Read the model definition and answer for the solid it produces. Units are mm, in the model's axes. A direction names the side the tool comes from. Coordinates: 2 decimals unless noted, no trailing zeros. Loops run counter-clockwise (first coordinate to the right, second up) from the corner with the lowest first, then second, coordinate; pieces in that order, holes last. Notation, with made-up numbers: (79.25, 29.25) -> (117.25, 29.25) arc R21 ccw to (117.25, 68.25) -> close; hole circle Ø7 at (-7, 74.5). An arc over 180 degrees is marked (long way). Answer as a JSON object with one key per item and string values. Group by question number.
Q1. The part is cut by section B-B on y = 0. Write down the section's boundary in (x, z).
Q2. The part is cut by section A-A on z = 4.3. Write down the section's boundary in (x, y).
Q3. For faces 1 (the flat face through (-9.754, 0, 4)), 2 (the cylindrical face through (-2.256, 0.154, 2.958)), determine the directions among +Z, -Z, +X, -X, +Y, -Y from which every point of the face is accessible in a straight line to the end or side of a thin tool.
Q4. Straight lines are drawn through the part: line 1 along Z through (x, y) = (-12.5, -1.5); line 2 along X through (y, z) = (4.25, 4.9); line 3 along X through (y, z) = (-3, 3.55). For each, find the intervals that lie inside material, in ascending order. Write a range as [from, to].
Q5. The part is cut by section D-D on y = 2.75. Write down the section's boundary in (x, z).
Q6. Determine the mould class of faces 3 (the cylindrical face through (-34.252, -0.154, 2.958)), 4 (the flat face through (-25.821, -5.446, 4.028)), 5 (the flat face through (-24, 0, 2)), 6 (the flat face through (-18.4, 7, 1.6)) for opening direction X: released by +X, released by -X, zero draft, split by the parting line, or undercut.
Q7. Each of these flat-tipped pins is pushed along its axis until it touches: P1, Ø1.5, axis at y = 5.5, z = 4, coming from the -X side; P2, Ø3, axis at y = 4.5, z = 4.5, coming from the -X side; P3, Ø1, axis at y = -2.5, z = 3, coming from the -X side. Where does it stop, or does it pass through?
Q8. The part is cut by section C-C on z = 1.25. Write down the section's boundary in (x, y), and give its area (3 significant figures).
from build123d import *
from OCP.BRepFilletAPI import BRepFilletAPI_MakeChamfer

# Parameters (mm, degrees)
BOSS_EXTRU_1_DEPTH      = 6
ESQUISSE3_R             = 5.5
ESQUISSE3_R_2           = 1.6
ENL_V_MAT_EXTRU_1_DEPTH = 36.47321166
ENL_V_MAT_EXTRU_2_DEPTH = 4
CHAMFER1_SIZE           = 2
CHAMFER1_SIZE2          = 1.464101615


with BuildPart() as part:
    # Esquisse1 → Boss.-Extru.1 (new body)
    with BuildSketch(Plane.XY):
        with BuildLine():
            Line((-27.254178511, 7), (-9.254178511, 7))
            ThreePointArc((-9.254178511, 7), (-2.254178511, 0), (-9.254178511, -7))
            Line((-9.254178511, -7), (-27.254178511, -7))
            ThreePointArc((-27.254178511, -7), (-34.254178511, 0), (-27.254178511, 7))
        make_face()
    extrude(amount=BOSS_EXTRU_1_DEPTH)

    # Esquisse3 → Enlèv. mat.-Extru.1 (cut, through all)
    with BuildSketch(Plane.XY.offset(6)):
        with Locations((-18.254178511, 0)):
            Circle(ESQUISSE3_R)
        with Locations((-30.254178511, 0)):
            Circle(ESQUISSE3_R_2)
        with Locations((-6.254178511, 0)):
            Circle(ESQUISSE3_R_2)
    extrude(amount=-ENL_V_MAT_EXTRU_1_DEPTH, mode=Mode.SUBTRACT)

    # Esquisse4 → Enlèv. mat.-Extru.2 (cut)
    with BuildSketch(Plane.XY.offset(6)):
        Polygon((-9.754178511, -4.907477288), (-9.754178511, 4.907477288), (-18.254178511, 9.814954576), (-26.754178511, 4.907477288), (-26.754178511, -4.907477288), (-18.254178511, -9.814954576), align=None)
    extrude(amount=-ENL_V_MAT_EXTRU_2_DEPTH, mode=Mode.SUBTRACT)

    # Chamfer1: one chamfer whose edges measure the first distance from different faces: ONE call of the kernel's chamfer builder (chamfer() names one face for all edges)
    chamfer1_edges_1 = [part.edges().sort_by_distance(p)[0] for p in [
        (-13.378534164, -7, 4),
    ]]
    chamfer1_side_1 = [part.faces().sort_by_distance(p)[0] for p in [
        (-11.566356337, -5.953738644, 4),
    ]]
    chamfer1_edges_2 = [part.edges().sort_by_distance(p)[0] for p in [
        (-23.129822858, -7, 4),
    ]]
    chamfer1_side_2 = [part.faces().sort_by_distance(p)[0] for p in [
        (-24.942000685, -5.953738644, 4),
    ]]
    chamfer1_edges_3 = [part.edges().sort_by_distance(p)[0] for p in [
        (-23.129822858, 7, 4),
    ]]
    chamfer1_side_3 = [part.faces().sort_by_distance(p)[0] for p in [
        (-24.942000685, 5.953738644, 4),
    ]]
    chamfer1_edges_4 = [part.edges().sort_by_distance(p)[0] for p in [
        (-13.378534164, 7, 4),
    ]]
    chamfer1_side_4 = [part.faces().sort_by_distance(p)[0] for p in [
        (-11.566356337, 5.953738644, 4),
    ]]
    chamfer1 = BRepFilletAPI_MakeChamfer(part.part.solid().wrapped)
    for e in chamfer1_edges_1:
        chamfer1.Add(CHAMFER1_SIZE, CHAMFER1_SIZE2, e.wrapped, chamfer1_side_1[0].wrapped)  # the first distance lies on this face
    for e in chamfer1_edges_2:
        chamfer1.Add(CHAMFER1_SIZE, CHAMFER1_SIZE2, e.wrapped, chamfer1_side_2[0].wrapped)  # the first distance lies on this face
    for e in chamfer1_edges_3:
        chamfer1.Add(CHAMFER1_SIZE, CHAMFER1_SIZE2, e.wrapped, chamfer1_side_3[0].wrapped)  # the first distance lies on this face
    for e in chamfer1_edges_4:
        chamfer1.Add(CHAMFER1_SIZE, CHAMFER1_SIZE2, e.wrapped, chamfer1_side_4[0].wrapped)  # the first distance lies on this face
    add(Compound.cast(chamfer1.Shape()), mode=Mode.REPLACE)


solid = part.part
Final values:
{
 "1": {"outline": "(-34.25, 0) -> (-31.85, 0) -> (-31.85, 6) -> (-34.25, 6) -> close; (-28.65, 0) -> (-23.75, 0) -> (-23.75, 2) -> (-26.75, 2) -> (-26.75, 6) -> (-28.65, 6) -> close; (-12.75, 0) -> (-7.85, 0) -> (-7.85, 6) -> (-9.75, 6) -> (-9.75, 2) -> (-12.75, 2) -> close; (-4.65, 0) -> (-2.25, 0) -> (-2.25, 6) -> (-4.65, 6) -> close"},
 "2": {"outline": "(-27.25, -7) -> (-24.59, -7) -> (-24.86, -6) -> (-26.75, -4.91) -> (-26.75, 4.91) -> (-24.86, 6) -> (-24.59, 7) -> (-27.25, 7) arc R7 ccw to start; (-11.91, -7) -> (-9.25, -7) arc R7 ccw to (-9.25, 7) -> (-11.91, 7) -> (-11.65, 6) -> (-9.75, 4.91) -> (-9.75, -4.91) -> (-11.65, -6) -> close; hole circle Ø3.2 at (-30.25, 0); hole circle Ø3.2 at (-6.25, 0)"},
 "3": {"face 1": "+Z", "face 2": "+Z, -Z, +X"},
 "4": {"line 1": "z = [0, 2]", "line 2": "x = [-32.82, -26.75], [-9.75, -3.69]", "line 3": "x = [-33.58, -26.75], [-9.75, -2.93]"},
 "5": {"outline": "(-33.69, 0) -> (-23.02, 0) -> (-23.02, 2) -> (-26.75, 2) -> (-26.75, 6) -> (-33.69, 6) -> close; (-13.49, 0) -> (-2.82, 0) -> (-2.82, 6) -> (-9.75, 6) -> (-9.75, 2) -> (-13.49, 2) -> close"},
 "6": {"face 3": "released by -X", "face 4": "undercut", "face 5": "undercut", "face 6": "zero draft"},
 "7": {"P1": "stops at x = -32.4", "P2": "stops at x = -33.58", "P3": "stops at x = -33.96"},
 "8": {"outline": "(-27.25, -7) -> (-9.25, -7) arc R7 ccw to (-9.25, 7) -> (-27.25, 7) arc R7 ccw to start; hole circle Ø3.2 at (-30.25, 0); hole circle Ø11 at (-18.25, 0); hole circle Ø3.2 at (-6.25, 0)", "area": "295 mm2"}
}
